CAD build for the part. Positions are in the model's coordinates, mm. A direction names the side the tool comes from. Round coordinates to 2 decimals unless told otherwise and drop trailing zeros. Loops run counter-clockwise (first coordinate to the right, second up) from the corner with the lowest first, then second, coordinate; pieces in that order, holes last. Notation, with made-up numbers: (-14.5, 84) - (35.5, 84) arc R14 cw to (35.5, 105) - close; hole circle Ø6 at (57, -1.75). An arc over 180 degrees is marked (long way). Use one line per item in the form item = value.
from build123d import *

# Parameters (mm, degrees)
SKETCH1_W                   = 30.408879848
SKETCH1_H                   = 29.21
SKETCH1_W_2                 = 11.358879848
SKETCH1_H_2                 = 5.08
BOSS_EXTRUDE1_DEPTH         = 5.08
F_1_4_0_25_DIAMETER_HOLE1_D = 6.35
SKETCH5_W                   = 13.97
SKETCH5_H                   = 29.21
BOSS_EXTRUDE2_DEPTH         = 5.08


with BuildPart() as part:
    # Sketch1 → Boss-Extrude1 (new body)
    with BuildSketch(Plane(origin=(0, 0, 0), x_dir=(1, 0, 0), z_dir=(0, 1, 0))):
        Rectangle(SKETCH1_W, SKETCH1_H)
        with Locations((0, 17.145)):
            Rectangle(SKETCH1_W_2, SKETCH1_H_2)
        with Locations((0, -17.145)):
            Rectangle(SKETCH1_W_2, SKETCH1_H_2)
    extrude(amount=BOSS_EXTRUDE1_DEPTH)

    # 1/4 (0.25) Diameter Hole1 (through all)
    with Locations(Plane(origin=(0, 5.08, 0), x_dir=(1, 0, 0), z_dir=(0, 1, 0))):
        with Locations((3.175, 0)):
            Hole(F_1_4_0_25_DIAMETER_HOLE1_D / 2)

    # Sketch5 → Boss-Extrude2 (add)
    with BuildSketch(Plane(origin=(0, 5.08, 0), x_dir=(1, 0, 0), z_dir=(0, 1, 0))):
        with Locations((22.189439924, 0)):
            Rectangle(SKETCH5_W, SKETCH5_H)
    extrude(amount=-BOSS_EXTRUDE2_DEPTH)


solid = part.part
1) Flat gauge pins, fed straight in: pin 1 (2.5 mm diameter, centred on y = 3.5, z = -17, fed in from +X); pin 2 (4 mm diameter, centred on x = 9, z = 6, fed in from -Y); pin 3 (1.5 mm diameter, centred on x = 14.5, y = 1, fed in from -Z) (3 decimals); pin 4 (1.5 mm diameter, centred on y = 2, z = 18.5, fed in from -X). Where does each tip first touch, or does it go through?
Report:
pin_1 = 5.68
pin_2 = 0
pin_3 = -14.605
pin_4 = -5.68
2) Slice it at A-A (z = 0). Write the cut outline in (x, y), plus the area to 3 significant figures.
Report:
outline = (-15.2, 0) - (0, 0) - (0, 5.08) - (-15.2, 5.08) - close; (6.35, 0) - (29.17, 0) - (29.17, 5.08) - (6.35, 5.08) - close
area = 193 mm^2
3) Slice it at B-B (y = 1.6). Write the cut outline in (x, z) (3 decimals).
Report:
outline = (-15.204, -14.605) - (-5.679, -14.605) - (-5.679, -19.685) - (5.679, -19.685) - (5.679, -14.605) - (29.174, -14.605) - (29.174, 14.605) - (5.679, 14.605) - (5.679, 19.685) - (-5.679, 19.685) - (-5.679, 14.605) - (-15.204, 14.605) - close; hole circle Ø6.35 at (3.175, 0)
4) Two-plate mould, pull along X, no slides. Class faces 1 (the flat face through (29.174, 3, 0)), 2 (the cylindrical face through (0.147, 2.504, -0.954)), 3 (the flat face through (-5.679, 3, -17)), 4 (the flat face through (0, 3, 19.685)): +X half, -X half, draft (parallel to the pull), parting line (faces both ways), or undercut.
Report:
face_1 = +X half
face_2 = undercut
face_3 = -X half
face_4 = draft
5) Tool access for faces 5 (the flat face through (-5.679, 3, 17)), 6 (the flat face through (-11, 3, -14.605)), 7 (the flat face through (5.679, 3, 17)): list every direction of +Z, -Z, +X, -X, +Y, -Y with a clear straight run to the whole face (end or side of a thin tool).
Report:
face_5 = +Z, -X, +Y, -Y
face_6 = -Z, -X, +Y, -Y
face_7 = +Z, +X, +Y, -Y
6) Slice it at D-D (z = -17). Write the cut outline in (x, y).
Report:
outline = (-5.68, 0) - (5.68, 0) - (5.68, 5.08) - (-5.68, 5.08) - close
7) Slice it at C-C (x = 24). Write the cut outline in (y, z) (3 decimals), plus the area to 3 significant figures.
Report:
outline = (0, -14.605) - (5.08, -14.605) - (5.08, 14.605) - (0, 14.605) - close
area = 148 mm^2
8) Drill centre lines: probe 1 along Z at (x, y) = (20, 3.4) (3 decimals); probe 2 along Z at (x, y) = (1, 4.2) (3 decimals); probe 3 along X at (y, z) = (3.45, 15.5). Where is each one in solid material? Low to high.
Report:
probe_1 = -14.605 to 14.605
probe_2 = -19.685 to -2.313, 2.313 to 19.685
probe_3 = -5.68 to 5.68
